Geometry check sheet. Reference: the model listing, model coordinates, mm. Give positions to 0.01 mm unless a question says otherwise; leave off trailing zeros. Loops run counter-clockwise (first coordinate to the right, second up) from the corner with the lowest first, then second, coordinate; pieces in that order, holes last.
1. Release check for a two-part mould opening along Y. For faces 1 (the cylindrical face through (-4.5, 4.6, 4.1)), 2 (the flat face through (16, 5, 8)), 3 (the cylindrical face through (33.847, 3.734, 4.056)) record: +Y half, -Y half, draft (parallel to the pull), parting line (faces both ways), or undercut.
2. Cross-section at C-C, the plane y = 6. Record the cut outline in (x, z), plus the area to 3 significant figures.
3. Material ranges on L1, parallel to X at y = 3, z = 2.25; L2, parallel to Y at x = 32, z = 4; L3, parallel to Y at x = 1.5, z = 2, recorded low to high.
4. Cross-section at A-A, the plane y = 4.5. Record the cut outline in (x, z).
5. Go/stop test with a flat-tipped pin: pin 1 Ø1 at (y, z) = (3.5, 1) entering from +X. Record where the tip stops, or that it passes through.
6. Cross-section at D-D, the plane y = 7.75. Record the cut outline in (x, z), plus the area to 3 significant figures.
7. Cross-section at B-B, the plane z = 6.25. Record the cut outline in (x, y).
from build123d import *

# Parameters (mm, degrees)
ESQUISSE1_W             = 32
ESQUISSE1_H             = 9
BOSS_EXTRU_1_DEPTH      = 8
BOSS_EXTRU_2_DEPTH      = 8
ESQUISSE3_R             = 2
ENL_V_MAT_EXTRU_1_DEPTH = 39.435010082


with BuildPart() as part:
    # Esquisse1 → Boss.-Extru.1 (new body)
    with BuildSketch(Plane.XY):
        with Locations((16, 4.5)):
            Rectangle(ESQUISSE1_W, ESQUISSE1_H)
    extrude(amount=BOSS_EXTRU_1_DEPTH)

    # Esquisse2 → Boss.-Extru.2 (add)
    with BuildSketch(Plane.XY.offset(8)):
        with BuildLine():
            Line((0, 0), (0, 9))
            ThreePointArc((0, 9), (-4.5, 4.5), (0, 0))
        make_face()
        with BuildLine():
            Line((32, 0), (32, 9))
            ThreePointArc((32, 9), (36.5, 4.5), (32, 0))
        make_face()
    extrude(amount=-BOSS_EXTRU_2_DEPTH)

    # Esquisse3 → Enlèv. mat.-Extru.1 (cut, through all)
    with BuildSketch(Plane.XY.offset(8)):
        with Locations((32, 4.5)):
            Circle(ESQUISSE3_R)
        with Locations((0, 4.5)):
            Circle(ESQUISSE3_R)
    extrude(amount=-ENL_V_MAT_EXTRU_1_DEPTH, mode=Mode.SUBTRACT)


solid = part.part
Result:
1. face 1: parting line
1. face 2: draft
1. face 3: undercut
2. outline: (-4.24, 0) - (-1.32, 0) - (-1.32, 8) - (-4.24, 8) - close; (1.32, 0) - (30.68, 0) - (30.68, 8) - (1.32, 8) - close; (33.32, 0) - (36.24, 0) - (36.24, 8) - (33.32, 8) - close
2. area: 282 mm2
3. L1: x = -4.24 to -1.32, 1.32 to 30.68, 33.32 to 36.24
3. L2: y = 0 to 2.5, 6.5 to 9
3. L3: y = 0 to 3.18, 5.82 to 9
4. outline: (-4.5, 0) - (-2, 0) - (-2, 8) - (-4.5, 8) - close; (2, 0) - (30, 0) - (30, 8) - (2, 8) - close; (34, 0) - (36.5, 0) - (36.5, 8) - (34, 8) - close
5. pin 1: stops at x = 36.47
6. outline: (-3.11, 0) - (35.11, 0) - (35.11, 8) - (-3.11, 8) - close
6. area: 306 mm2
7. outline: (0, 0) - (32, 0) arc R4.5 ccw to (32, 9) - (0, 9) arc R4.5 ccw to start; hole circle Ø4 at (0, 4.5); hole circle Ø4 at (32, 4.5)
